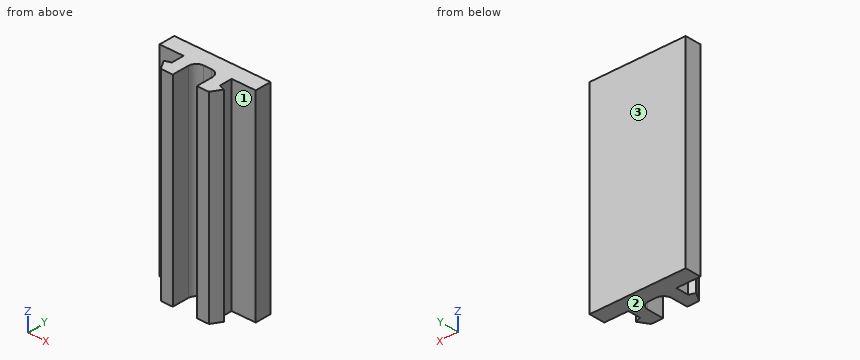
```python
from build123d import *

# Parameters (mm, degrees)
BOSS_EXTRUDE1_DEPTH = 25


with BuildPart() as part:
    # Sketch1 → Boss-Extrude1 (new body)
    with BuildSketch(Plane.XY):
        with BuildLine():
            Line((0, 0), (12, 0))
            Line((12, 0), (12, -2))
            Line((12, -2), (9, -2))
            Line((9, -2), (9, -3.6))
            Line((9, -3.6), (9.751754097, -3.873616115))
            Line((9.751754097, -3.873616115), (9, -5.1))
            Line((9, -5.1), (7.5, -5.1))
            Line((7.5, -5.1), (7.5, -3))
            ThreePointArc((7.5, -3), (7.207106781, -2.292893219), (6.5, -2))
            Line((6.5, -2), (5.5, -2))
            ThreePointArc((5.5, -2), (4.792893219, -2.292893219), (4.5, -3))
            Line((4.5, -3), (4.5, -5.1))
            Line((4.5, -5.1), (3, -5.1))
            Line((3, -5.1), (2.248245903, -3.873616115))
            Line((2.248245903, -3.873616115), (3, -3.6))
            Line((3, -3.6), (3, -2))
            Line((3, -2), (0, -2))
            Line((0, -2), (0, 0))
        make_face()
    extrude(amount=BOSS_EXTRUDE1_DEPTH)


solid = part.part
```
Verification items for the finished model (mm, model axes). Face numbers are marked on the shaded views. Give positions to 0.01 mm unless a question says otherwise; leave off trailing zeros. Order: outer loops, then holes, each group sorted by start corner. A loop starts at its lowest first (then second) coordinate and runs counter-clockwise, first axis right, second up. Notation, with made-up numbers: (-38.5, 32) -> (15.5, 32) arc R10 ccw to (15.5, 45) -> close; hole circle Ø9 at (-6, 53). An arc over 180 degrees is marked (long way). Use a Markdown table: item, result.
1) Section check A-A, the plane y = -4.25. Record the boundary of the cut face in (x, z).
Results:
| item | result |
|---|---|
| outline | (2.48, 0) -> (4.5, 0) -> (4.5, 25) -> (2.48, 25) -> close; (7.5, 0) -> (9.52, 0) -> (9.52, 25) -> (7.5, 25) -> close |
2) Section check C-C, the plane y = -2.5. Record the boundary of the cut face in (x, z), then the cut area to 3 significant figures.
Results:
| item | result |
|---|---|
| outline | (3, 0) -> (4.63, 0) -> (4.63, 25) -> (3, 25) -> close; (7.37, 0) -> (9, 0) -> (9, 25) -> (7.37, 25) -> close |
| area | 81.7 mm² |
3) Section check D-D, the plane x = 10.75. Record the boundary of the cut face in (y, z), then the cut area to 3 significant figures.
Results:
| item | result |
|---|---|
| outline | (-2, 0) -> (0, 0) -> (0, 25) -> (-2, 25) -> close |
| area | 50.0 mm² |
4) Depth check by flat-ended pin: pin 1 Ø0.8 at (y, z) = (-3, 8) entering from -X; pin 2 Ø2.5 at (x, z) = (10.5, 10.5) entering from -Y; pin 3 Ø0.9 at (x, z) = (1, 17) entering from -Y. Enter the tip coordinate at first touch or a pass-through.
Results:
| item | result |
|---|---|
| pin 1 | x = 3 |
| pin 2 | y = -4.69 |
| pin 3 | y = -2 |
5) Material ranges on probe 1 along X at (y, z) = (-3.25, 20.75); probe 2 along Y at (x, z) = (6, 13.75); probe 3 along X at (y, z) = (-2.2, 16.5), recorded low to high.
Results:
| item | result |
|---|---|
| probe 1 | 3 to 4.5, 7.5 to 9 |
| probe 2 | -2 to 0 |
| probe 3 | 3 to 4.9, 7.1 to 9 |
6) Mould release check, pull along Y, two halves, no side actions. Record for the marked faces 1, 2 and 3: pulls with the +Y half, pulls with the -Y half, needs draft (parallel to the pull), parting line crosses it, or undercut.
Results:
| item | result |
|---|---|
| face 1 | undercut |
| face 2 | needs draft |
| face 3 | pulls with the +Y half |
7) Section check B-B, the plane z = 11. Record the boundary of the cut face in (x, y).
Results:
| item | result |
|---|---|
| outline | (0, -2) -> (3, -2) -> (3, -3.6) -> (2.25, -3.87) -> (3, -5.1) -> (4.5, -5.1) -> (4.5, -3) arc R1 cw to (5.5, -2) -> (6.5, -2) arc R1 cw to (7.5, -3) -> (7.5, -5.1) -> (9, -5.1) -> (9.75, -3.87) -> (9, -3.6) -> (9, -2) -> (12, -2) -> (12, 0) -> (0, 0) -> close |
